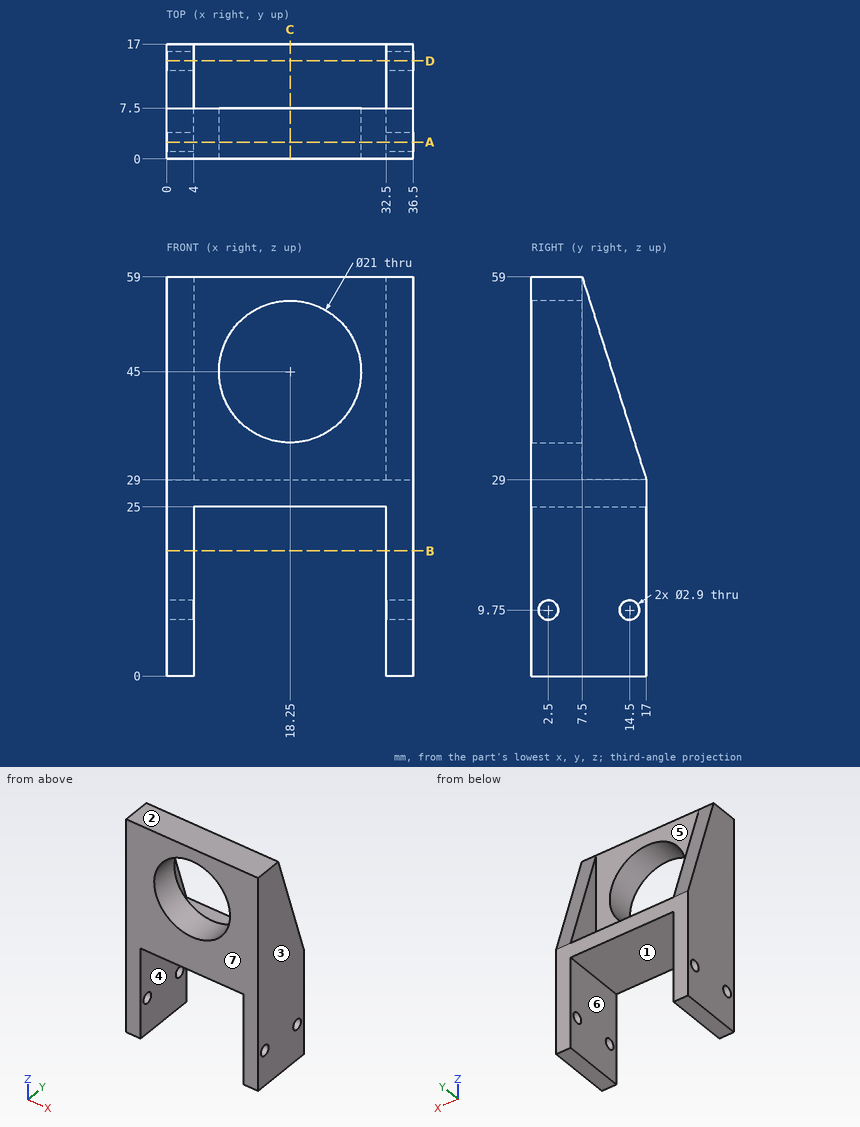
Geometry: see drawing. Coordinates: mm, zero at the bounding-box minimum. A direction names the side the tool comes from. Give positions to 0.01 mm unless a question says otherwise; leave off trailing zeros. Loops run counter-clockwise (first coordinate to the right, second up) from the corner with the lowest first, then second, coordinate; pieces in that order, holes last. Notation, with made-up numbers: M 77.25,26 L 82.25,26 A36 ccw 82.25,61 Z; hole C 74,54 d6. An arc over 180 degrees is marked long. Use one line per item in the form item = value.
1. Section query D-D, the plane y = 14.5. Return the cut outline in (x, z), and give its area (3 significant figures).
Numbers:
outline = M 0,0 L 4,0 L 4,8.3 L 0,8.3 Z; M 0,11.2 L 4,11.2 L 4,25 L 32.5,25 L 32.5,11.2 L 36.5,11.2 L 36.5,36.89 L 32.5,36.89 L 32.5,29 L 4,29 L 4,36.89 L 0,36.89 Z; M 32.5,0 L 36.5,0 L 36.5,8.3 L 32.5,8.3 Z
area = 386 mm²
2. Section query C-C, the plane x = 18.25. Return the cut outline in (y, z), and give its area (4 significant figures).
Numbers:
outline = M 0,25 L 17,25 L 17,29 L 7.5,29 L 7.5,34.5 L 0,34.5 Z; M 0,55.5 L 7.5,55.5 L 7.5,59 L 0,59 Z
area = 135.5 mm²
3. Pull-direction query (X, two-part tool) for the marked faces 1, 2, 3 and 4; classes: released by +X, released by -X, zero draft, split by the parting line, or undercut.
Numbers:
face_1 = undercut
face_2 = zero draft
face_3 = released by +X
face_4 = undercut
4. Section query A-A, the plane y = 2.5. Return the cut outline in (x, z).
Numbers:
outline = M 0,0 L 4,0 L 4,8.3 L 0,8.3 Z; M 0,11.2 L 4,11.2 L 4,25 L 32.5,25 L 32.5,11.2 L 36.5,11.2 L 36.5,59 L 0,59 Z; M 32.5,0 L 36.5,0 L 36.5,8.3 L 32.5,8.3 Z; hole C 18.25,45 d21
5. Section query B-B, the plane z = 18.5. Return the cut outline in (x, y), and give its area (3 significant figures).
Numbers:
outline = M 0,0 L 4,0 L 4,17 L 0,17 Z; M 32.5,0 L 36.5,0 L 36.5,17 L 32.5,17 Z
area = 136 mm²
6. Reachability of the marked faces 5, 6 and 7 from +Z, -Z, +X, -X, +Y, -Y: full face, straight path, thin tool, end or side. Return the list, or none.
Numbers:
face_5 = +Z, +Y
face_6 = -Z, +Y, -Y
face_7 = +Z, -Z, +X, -X, -Y
7. First-contact query: pin 1 (3 mm diameter, centred on x = 22, y = 12.5, fed in from +Z); pin 2 (8 mm diameter, centred on x = 28, y = 13.5, fed in from -Z); pin 3 (1.7 mm diameter, centred on y = 2.5, z = 9.75, fed in from -X). Flat tips, straight axial feed; report the tip coordinate or a pass-through.
Numbers:
pin_1 = 29
pin_2 = 25
pin_3 = through
8. Line query: L1, parallel to Y at x = 3.2, z = 9.75; L2, parallel to Z at x = 3.05, y = 2.5; L3, parallel to X at y = 3.5, z = 45. Output: solid intervals per line, ascending.
Numbers:
L1 = 0 to 1.05, 3.95 to 13.05, 15.95 to 17
L2 = 0 to 8.3, 11.2 to 59
L3 = 0 to 7.75, 28.75 to 36.5
